```python
from build123d import *

# Parameters (mm, degrees)
SKETCH1_R           = 30
BOSS_EXTRUDE1_DEPTH = 3
SKETCH1_3_R         = 6
SKETCH1_3_R_2       = 4.1
BOSS_EXTRUDE2_DEPTH = 10
BOSS_EXTRUDE3_DEPTH = 10
CIRPATTERN4_COUNT   = 3


with BuildPart() as part:
    # Sketch1 → Boss-Extrude1 (new body)
    with BuildSketch(Plane(origin=(0, 0, 0), x_dir=(1, 0, 0), z_dir=(0, 1, 0))):
        with Locations(Location((0, 0, 0), (0, 0, 270))):
            Circle(SKETCH1_R)
    extrude(amount=-BOSS_EXTRUDE1_DEPTH)

    # Sketch1_3 → Boss-Extrude2 (add)
    with BuildSketch(Plane(origin=(0, 0, 0), x_dir=(1, 0, 0), z_dir=(0, 1, 0))):
        with Locations(Location((0, 0, 0), (0, 0, 270))):
            Circle(SKETCH1_3_R)
        with Locations(Location((0, 0, 0), (0, 0, 270))):
            Circle(SKETCH1_3_R_2, mode=Mode.SUBTRACT)
    extrude(amount=BOSS_EXTRUDE2_DEPTH)

    # Sketch3 → Boss-Extrude3 (add, symmetric)
    with BuildSketch(Plane.XY):
        with BuildLine():
            Line((20.986182934, 0), (20.986182934, 1))
            Line((20.986182934, 1), (30, 1))
            add(Edge.make_bspline(
                [(30, 1), (60.374034606, 1), (76.330152451, -22.351113915), (80.195520174, -45.635895635)],
                knots=[0, 0, 0, 0, 1, 1, 1, 1], degree=3))
            Line((80.195520174, -45.635895635), (79.209020453, -45.799658569))
            add(Edge.make_bspline(
                [(30.99996266, -0.008641626), (31.899242715, -0.024239786), (33.715729703, -0.099542856), (37.190019089, -0.416822027), (41.343618956, -1.117068291), (45.997769292, -2.40892623), (51.783186603, -4.689972725), (58.237135031, -8.508276888), (64.779288573, -14.388068011), (70.145770006, -21.31599418), (74.357167494, -29.037194285), (76.919217392, -35.910251352), (78.412064798, -41.54676245), (78.972472907, -44.374707991), (79.209020453, -45.799658569)],
                knots=[0.011223961, 0.011223961, 0.011223961, 0.011223961, 0.042123212, 0.073022463, 0.134820966, 0.196619468, 0.258417971, 0.382014975, 0.50561198, 0.629208985, 0.75280599, 0.876402995, 0.938201498, 1, 1, 1, 1], degree=3))
            Line((30.99996266, -0.008641626), (20.986182934, 0))
        make_face()
    boss_extrude3 = extrude(amount=BOSS_EXTRUDE3_DEPTH, both=True)

    # CirPattern4: Boss-Extrude3 ×3 about axis
    cirpattern4_axis = Axis((0, 10, 0), (0, -1, 0))
    for i in range(1, CIRPATTERN4_COUNT):
        add(boss_extrude3.rotate(cirpattern4_axis, i * 360 / CIRPATTERN4_COUNT))


solid = part.part
```
Check sheet for the modelled part. Datum: model origin and axes. Units: mm. A direction names the side the tool comes from. Give positions to 0.01 mm unless a question says otherwise; leave off trailing zeros. Write each loop counter-clockwise with the first axis right and the second up, starting at its lowest first coordinate (ties: lowest second). Pieces come first, ordered by that corner, then holes. Notation, with made-up numbers: (9, 49.5) -> (43, 49.5) arc R29 ccw to (43, 84.5) -> close; hole circle Ø8 at (-18, -10.75). An arc over 180 degrees is marked (long way). Use CSV: the item, a comma, the result in double quotes. Start each with the question number.
Q1. Cross-section at B-B on x = 0. Enter the section's corners in (y, z).
Q2. Depth check by flat-ended pin: P1, Ø12, axis at y = -23, z = 4.5, coming from the +X side; P2, Ø13, axis at x = 0, z = 0, coming from the -Y side; P3, Ø9, axis at x = -13.5, z = 19.5, coming from the +Y side. Enter the tip coordinate at first touch or a pass-through.
Q3. Release check for a two-part mould opening along X. For faces 4 (the flat face through (0, 0, 0)), 5 (the flat face through (-35.12, -4.96, -40.83)), 6 (the flat face through (0, -3, 0)), 7 (the cylindrical face through (1.32, -1.48, -29.97)) record: +X half, -X half, draft (parallel to the pull), parting line (faces both ways), or undercut.
Q4. Cross-section at C-C on y = -25. Count the separate pieces of the cut face and the enclosed holes in it, and give its area (3 significant figures).
Q5. Tool access check on faces 1 (the flat face through (-17.8, -4.96, 50.83)), 2 (the cylindrical face through (1.802, 4.93, 5.723)), 3 (the flat face through (-35.12, -4.96, 40.83)). Record the directions out of +Z, -Z, +X, -X, +Y, -Y that give a thin tool (end or side, any length) a straight path to the whole face; none if there is none.
Q6. Scan lines: line 1 along X through (y, z) = (3, 0); line 2 along Z through (x, y) = (-38.5, -42.5); line 3 along Z through (x, y) = (-20, -7). Record each from-to range of solid material in increasing order.
Q7. Cross-section at A-A on y = 6. Enter the section's corners in (x, z).
Working result:
1,outline,"(-3, -30) -> (0, -30) -> (0, -6) -> (10, -6) -> (10, -4.1) -> (0, -4.1) -> (0, 4.1) -> (10, 4.1) -> (10, 6) -> (0, 6) -> (0, 30) -> (-3, 30) -> close"
2,P1,"stops at x = 75.21"
2,P2,"stops at y = -3"
2,P3,"stops at y = 1"
3,face 4,"undercut"
3,face 5,"-X half"
3,face 6,"draft"
3,face 7,"undercut"
4,separate pieces,"3"
4,enclosed holes,"0"
4,area,"68.4 mm^2"
5,face 1,"+Z, +X, +Y"
5,face 2,"+Y"
5,face 3,"-X, +Y"
6,line 1,"x = -6 to -4.1, 4.1 to 6"
6,line 2,"z = -69.69 to -68.51, 68.51 to 69.69"
6,line 3,"z = -54.64 to -52.54, 52.54 to 54.64"
7,outline,"circle Ø12 at (0, 0); hole circle Ø8.2 at (0, 0)"
